```python
from build123d import *

# Parameters (mm, degrees)
F0_W     = 19.05
F0_H     = 19.05
F1_DEPTH = 9.525
F5_R     = 3.96875
F6_DEPTH = 9.525
F9_DEPTH = 19.05


with BuildPart() as f1:
    # F0 (on Front) → F1 (new body)
    with BuildSketch(Plane.XZ):
        Rectangle(F0_W, F0_H)
    extrude(amount=F1_DEPTH)

    # F3 (on Right) → F4 (revolve, cut)
    with BuildSketch(Plane.YZ):
        Polygon((-2.8980535523, 20.3406831001), (0, 9.525), (0, 20.3406831001), align=None)
    revolve(axis=Axis((0, 0, 0), (0, 1, 0)), mode=Mode.SUBTRACT)

    # F5 (on face) → F6 (cut)
    with BuildSketch(Plane(origin=(0, 0, 0), x_dir=(-1, 0, 0), z_dir=(0, 1, 0))):
        Circle(F5_R)
    extrude(amount=-F6_DEPTH, mode=Mode.SUBTRACT)

    # F7: F1 across face


with BuildPart() as f1_1:
    add(f1.part)
    add(f1.part.mirror(Plane.XZ.offset(9.525)))

    # F8 (on face) → F9 (cut)
    with BuildSketch(Plane(origin=(-9.525, 0, 0), x_dir=(0, -1, 0), z_dir=(-1, 0, 0))):
        Polygon((8.4074, 9.525), (9.525, 8.4074), (10.6426, 9.525), align=None)
    extrude(amount=-F9_DEPTH, mode=Mode.SUBTRACT)


solid = f1_1.part
```
Part model, mm, in its own coordinate system. A direction names the side the tool comes from. Round coordinates to 2 decimals unless told otherwise and drop trailing zeros. Loops run counter-clockwise (first coordinate to the right, second up) from the corner with the lowest first, then second, coordinate; pieces in that order, holes last.
1. Two-plate mould, pull along Y, no slides. Class faces 3 (the face through (-0.13, -8.96, 8.97)), 4 (the face through (-7.37, -0.25, -7.43)), 5 (the face through (9.525, -10, 0)): pulls with the +Y half, pulls with the -Y half, needs draft (parallel to the pull), parting line crosses it, or undercut.
Solutions:
face 3: undercut
face 4: pulls with the +Y half
face 5: needs draft
2. Slice it at A-A (y = -3.75). Give the cut face in (x, z) (1 decimal).
Solutions:
outline: (-9.5, -9.5) - (9.5, -9.5) - (9.5, 9.5) - (-9.5, 9.5) - close; hole circle Ø7.9 at (0, 0)
3. Drill centre lines: line 1 along Z through (x, y) = (1.5, -4.25) (3 decimals); line 2 along Y through (x, z) = (8.5, 6.75). Where is each one in solid material? Low to high.
Solutions:
line 1: z = -9.525 to -3.674, 3.674 to 9.525
line 2: y = -18.69 to -0.36
4. 3-axis set-ups, long thin cutter, end or side, ignore diameter. For faces 1 (the face through (-0.13, -10.08, 8.96)), 2 (the face through (4, 0, -2)): which of +Z, -Z, +X, -X, +Y, -Y reach the whole face in a straight line?
Solutions:
face 1: +Z, +X, -X
face 2: +Z, -Z, +X, -X, +Y
